Part model, mm, in its own coordinate system. A direction names the side the tool comes from. Coordinates: 2 decimals unless noted, no trailing zeros. Loops run counter-clockwise (first coordinate to the right, second up) from the corner with the lowest first, then second, coordinate; pieces in that order, holes last. Notation, with made-up numbers: M -38,27.25 L -19,27.25 A27 cw -19,58.25 Z; hole C 53,13.25 d7. An arc over 180 degrees is marked long. Answer as a JSON object with one key per item and string values. Group by question number.
1. 3-axis set-ups, long thin cutter, end or side, ignore diameter. For faces 1 (the face through (-28, 30, 0)), 2 (the face through (-27.85, -27.01, -1.97)): which of +Z, -Z, +X, -X, +Y, -Y reach the whole face in a straight line?
2. Saw through at B-B on x = -31. Write the cut outline in (y, z).
3. Saw through at A-A on y = -28. Write the cut outline in (x, z), then the cut area to 3 significant figures.
4. Saw through at C-C on z = -0.75. Write the cut outline in (x, y), then the cut area to 3 significant figures.
5. Drop flat-ended pins along their axis: pin 1 Ø1.5 at (x, z) = (-30, 1) entering from -Y; pin 2 Ø7 at (x, y) = (-22.5, -29.5) entering from +Z; pin 3 Ø1.5 at (x, z) = (-21.5, 1) entering from +Y. Give the stop position or say it passes through.
6. Drill centre lines: L1, parallel to Y at x = -31, z = -2.8; L2, parallel to Z at x = -39.5, y = -32; L3, parallel to Y at x = -40.5, z = 2.5. Where is each one in solid material? Low to high.
7. Saw through at D-D on x = -24. Write the cut outline in (y, z).
8. Mould opens along Y. For faces 3 (the face through (-28, -21, 1)), 4 (the face through (-28, -26, 0)), 5 (the face through (-27.95, 26.74, -1.97)) say: released by +Y, released by -Y, zero draft, split by the parting line, or undercut.
from build123d import *

# Parameters (mm, degrees)
F0_W     = 55
F0_H     = 14
F0_R     = 3.3
F0_H_2   = 42
F1_DEPTH = 4
F2_DEPTH = 3


with BuildPart() as f1:
    # F0 (on Top) → F1 (new body)
    with BuildSketch(Plane.XY):
        with Locations((-27.5, 28)):
            Rectangle(F0_W, F0_H)
        with Locations((-31, 28)):
            Circle(F0_R, mode=Mode.SUBTRACT)
        with Locations((-27.5, 0)):
            Rectangle(F0_W, F0_H_2)
        with Locations((-27.5, -28)):
            Rectangle(F0_W, F0_H)
        with Locations((-31, -28)):
            Circle(F0_R, mode=Mode.SUBTRACT)
    extrude(amount=-F1_DEPTH)

    # F0 (on Top) → F2 (join)
    with BuildSketch(Plane.XY):
        with Locations((-27.5, 0)):
            Rectangle(F0_W, F0_H_2)
    extrude(amount=F2_DEPTH)


solid = f1.part
Outcome:
{
 "1": {"face 1": "+Z, +X, -X, +Y", "face 2": "+Z, -Z"},
 "2": {"outline": "M -35,-4 L -31.3,-4 L -31.3,0 L -35,0 Z; M -24.7,-4 L 24.7,-4 L 24.7,0 L 21,0 L 21,3 L -21,3 L -21,0 L -24.7,0 Z; M 31.3,-4 L 35,-4 L 35,0 L 31.3,0 Z"},
 "3": {"outline": "M -55,-4 L -34.3,-4 L -34.3,0 L -55,0 Z; M -27.7,-4 L 0,-4 L 0,0 L -27.7,0 Z", "area": "194 mm²"},
 "4": {"outline": "M -55,-35 L 0,-35 L 0,35 L -55,35 Z; hole C -31,-28 d6.6; hole C -31,28 d6.6", "area": "3,780 mm²"},
 "5": {"pin 1": "stops at y = -21", "pin 2": "stops at z = 0", "pin 3": "stops at y = 21"},
 "6": {"L1": "y = -35 to -31.3, -24.7 to 24.7, 31.3 to 35", "L2": "z = -4 to 0", "L3": "y = -21 to 21"},
 "7": {"outline": "M -35,-4 L 35,-4 L 35,0 L 21,0 L 21,3 L -21,3 L -21,0 L -35,0 Z"},
 "8": {"face 3": "released by -Y", "face 4": "zero draft", "face 5": "undercut"}
}
